The model under review builds one solid part; all positions refer to its coordinate system, in mm. A direction names the side the tool comes from. Round coordinates to 2 decimals unless told otherwise and drop trailing zeros. Loops run counter-clockwise (first coordinate to the right, second up) from the corner with the lowest first, then second, coordinate; pieces in that order, holes last. Notation, with made-up numbers: M 78,24 L 123,24 A27 cw 123,41 Z; hole C -40,14.25 d10. An arc over 180 degrees is marked long. One line per question, with ' | ' between items.
from build123d import *

# Parameters (mm, degrees)
SKETCH1_R           = 50.25
BOSS_EXTRUDE1_DEPTH = 53.5
SKETCH2_R           = 50.5
CUT_EXTRUDE1_DEPTH  = 31
SKETCH3_R           = 27.5
BOSS_EXTRUDE2_DEPTH = 13.5
SKETCH8_R           = 15.5
BOSS_EXTRUDE4_DEPTH = 5
SKETCH9_R           = 2
CUT_EXTRUDE5_DEPTH  = 115.494541355
SKETCH10_R          = 22.5
CUT_EXTRUDE6_DEPTH  = 1


with BuildPart() as part:
    # Sketch1 → Boss-Extrude1 (new body)
    with BuildSketch(Plane.XY):
        with BuildLine():
            Line((-55, 43.301270189), (-55, -43.301270189))
            ThreePointArc((-55, -43.301270189), (0, -70), (55, -43.301270189))
            Line((55, -43.301270189), (55, 43.301270189))
            ThreePointArc((55, 43.301270189), (0, 70), (-55, 43.301270189))
        make_face()
        Circle(SKETCH1_R, mode=Mode.SUBTRACT)
    extrude(amount=BOSS_EXTRUDE1_DEPTH)

    # Sketch2 → Cut-Extrude1 (cut)
    with BuildSketch(Plane.XY.offset(53.5)):
        Circle(SKETCH2_R)
    extrude(amount=-CUT_EXTRUDE1_DEPTH, mode=Mode.SUBTRACT)

    # Sketch3 → Boss-Extrude2 (add)
    with BuildSketch(Plane.XY.offset(53.5)):
        with BuildLine():
            Line((-55, -43.301270189), (-55, 43.301270189))
            ThreePointArc((-55, 43.301270189), (0, 70), (55, 43.301270189))
            Line((55, 43.301270189), (55, -43.301270189))
            ThreePointArc((55, -43.301270189), (0, -70), (-55, -43.301270189))
        make_face()
        Circle(SKETCH3_R, mode=Mode.SUBTRACT)
    extrude(amount=BOSS_EXTRUDE2_DEPTH)

    # Sketch8 → Boss-Extrude4 (add)
    with BuildSketch(Plane.XY.offset(67)):
        with BuildLine():
            Line((-55, 43.301270189), (-55, -43.301270189))
            ThreePointArc((-55, -43.301270189), (0, -70), (55, -43.301270189))
            Line((55, -43.301270189), (55, 43.301270189))
            ThreePointArc((55, 43.301270189), (0, 70), (-55, 43.301270189))
        make_face()
        Circle(SKETCH8_R, mode=Mode.SUBTRACT)
    extrude(amount=BOSS_EXTRUDE4_DEPTH)

    # Sketch9 → Cut-Extrude5 (cut, through all)
    with BuildSketch(Plane.XY.offset(72)):
        with Locations((-35, -48.733971724)):
            Circle(SKETCH9_R)
        with Locations((-35, 48.733971724)):
            Circle(SKETCH9_R)
        with Locations((35, 48.733971724)):
            Circle(SKETCH9_R)
        with Locations((35, -48.733971724)):
            Circle(SKETCH9_R)
    extrude(amount=-CUT_EXTRUDE5_DEPTH, mode=Mode.SUBTRACT)

    # Sketch10 → Cut-Extrude6 (cut)
    with BuildSketch(Plane(origin=(0, 0, 67), x_dir=(-1, 0, 0), z_dir=(0, 0, -1))):
        Circle(SKETCH10_R)
    extrude(amount=-CUT_EXTRUDE6_DEPTH, mode=Mode.SUBTRACT)


solid = part.part
1) Add section D-D on x = 35. State the section outline as (y, z) points.
Output values:
outline: M -60.62,0 L -50.73,0 L -50.73,72 L -60.62,72 Z; M -46.73,0 L -36.06,0 L -36.06,22.5 L -36.4,22.5 L -36.4,53.5 L 36.4,53.5 L 36.4,22.5 L 36.06,22.5 L 36.06,0 L 46.73,0 L 46.73,72 L -46.73,72 Z; M 50.73,0 L 60.62,0 L 60.62,72 L 50.73,72 Z
2) Machinability: for faces 4 (the cylindrical face through (-10.95, -49.3, 38.22)), 5 (the cylindrical face through (-10.382, -19.961, 67.493)), 6 (the flat face through (-21, -46, 0)), which of the approach directions +Z, -Z, +X, -X, +Y, -Y give a long, thin tool a straight path to every point of the face, cutting with its end or side? Answer none if there is none.
Output values:
face 4: none | face 5: -Z | face 6: -Z, +X, -X, +Y, -Y
3) Mouldability with a two-part tool opening along X and no side actions: class faces 1 (the flat face through (-15, 5, 68)), 2 (the cylindrical face through (-0.886, -69.994, 35.496)), 3 (the flat face through (-1, 17, 72)) as +X half, -X half, draft (parallel to the pull), parting line (faces both ways), or undercut.
Output values:
face 1: undercut | face 2: parting line | face 3: draft
4) Insertion check: P1, Ø10, axis at x = 37.5, z = 64, coming from the -Y side; P2, Ø12, axis at x = -13.5, z = 47.5, coming from the -Y side; P3, Ø1, axis at x = -2, z = 62.5, coming from the +Y side; P4, Ø25, axis at x = 0, y = 0, coming from the -Z side. Each pin has a flat end and moves straight along its axis. Give the tip position at first contact, or say it passes through.
Output values:
P1: stops at y = -62 | P2: stops at y = -69.6 | P3: stops at y = 69.98 | P4: passes through
5) Add section B-B on x = 0. State the section outline as (y, z) points, then the cut area to 3 significant figures.
Output values:
outline: M -70,0 L -50.25,0 L -50.25,22.5 L -50.5,22.5 L -50.5,53.5 L -27.5,53.5 L -27.5,67 L -22.5,67 L -22.5,68 L -15.5,68 L -15.5,72 L -70,72 Z; M 15.5,68 L 22.5,68 L 22.5,67 L 27.5,67 L 27.5,53.5 L 50.5,53.5 L 50.5,22.5 L 50.25,22.5 L 50.25,0 L 70,0 L 70,72 L 15.5,72 Z | area: 3,780 mm²
6) Add section C-C on z = 20. State the section outline as (x, y) points.
Output values:
outline: M -55,-43.3 A70 ccw 55,-43.3 L 55,43.3 A70 ccw -55,43.3 Z; hole C 0,0 d100.5; hole C -35,-48.73 d4; hole C -35,48.73 d4; hole C 35,-48.73 d4; hole C 35,48.73 d4
7) Add section A-A on y = 0. State the section outline as (x, z) points.
Output values:
outline: M -55,0 L -50.25,0 L -50.25,22.5 L -50.5,22.5 L -50.5,53.5 L -27.5,53.5 L -27.5,67 L -22.5,67 L -22.5,68 L -15.5,68 L -15.5,72 L -55,72 Z; M 15.5,68 L 22.5,68 L 22.5,67 L 27.5,67 L 27.5,53.5 L 50.5,53.5 L 50.5,22.5 L 50.25,22.5 L 50.25,0 L 55,0 L 55,72 L 15.5,72 Z
8) For line 1 (X direction, y = 0, z = 16); line 2 (X direction, y = 0, z = 69); line 3 (Y direction, x = 35, z = 19), list the stretches that pass through material, from the lowest coordinate up.
Output values:
line 1: x = -55 to -50.25, 50.25 to 55 | line 2: x = -55 to -15.5, 15.5 to 55 | line 3: y = -60.62 to -50.73, -46.73 to -36.06, 36.06 to 46.73, 50.73 to 60.62
